The listing builds one solid part. Answer for the finished solid, in the listing's coordinates (mm). Coordinates: 2 decimals unless noted, no trailing zeros. Order: outer loops, then holes, each group sorted by start corner. A loop starts at its lowest first (then second) coordinate and runs counter-clockwise, first axis right, second up. Notation, with made-up numbers: M 14.5,-38.75 L 33.5,-38.75 A13 ccw 33.5,-22.75 Z; hole C 66.25,-25 d8. An arc over 180 degrees is marked long. One line per item, written item: value. Start each with the question number.
Q1. This flat-tipped pin is pushed along its axis until it touches: pin 1 Ø5.5 at (x, y) = (0, 60) entering from +Z. Where does it stop, or does it pass through?
Q2. Straight lines are drawn through the part: line 1 along Y through (x, z) = (0, 0.4); line 2 along Y through (x, z) = (2, 0.95); line 3 along X through (y, z) = (22.5, 1.15). For each, find the intervals that lie inside material, in ascending order. Write a range as [from, to].
Q3. The part is cut by section B-B on z = 1.3. Give the vertices of the cut face in (x, y), then the cut area to 3 significant figures.
Q4. The part is cut by section D-D on y = -62. Give the vertices of the cut face in (x, z).
Q5. The part is cut by section A-A on x = 0. Give the vertices of the cut face in (y, z), then the cut area to 3 significant figures.
Q6. The part is cut by section C-C on y = 60. Give the vertices of the cut face in (x, z), then the cut area to 3 significant figures.
```python
from build123d import *

# Parameters (mm, degrees)
SKETCH_1_W        = 40
SKETCH_1_H        = 160
EXTRUDE_1_DEPTH   = 2
CHAMFER_1_SIZE    = 2
HOLE_WIZARD_M81_D = 9


with BuildPart() as part:
    # Эскиз1 → Бобышка-Вытянуть1 (new body)
    with BuildSketch(Plane.XY):
        Rectangle(SKETCH_1_W, SKETCH_1_H)
    extrude(amount=EXTRUDE_1_DEPTH)

    # Фаска1
    chamfer_1_edges = [part.edges().sort_by_distance(p)[0] for p in [
        (20, -80, 1),
        (-20, -80, 1),
        (-20, 80, 1),
        (20, 80, 1),
    ]]
    chamfer(chamfer_1_edges, length=CHAMFER_1_SIZE)

    # Отверстие с зазором M81 (through all)
    with Locations(Plane.XY.offset(2)):
        with Locations((0, -60), (0, 60), (0, 20), (0, -20)):
            Hole(HOLE_WIZARD_M81_D / 2)


solid = part.part
```
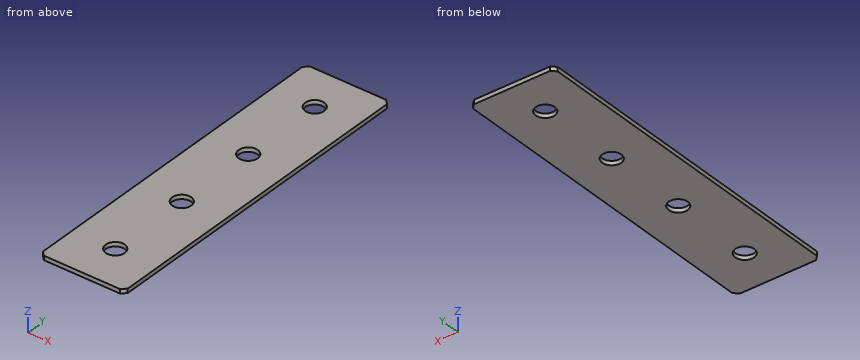
Output:
1. pin 1: passes through
2. line 1: y = [-80, -64.5], [-55.5, -24.5], [-15.5, 15.5], [24.5, 55.5], [64.5, 80]
2. line 2: y = [-80, -64.03], [-55.97, -24.03], [-15.97, 15.97], [24.03, 55.97], [64.03, 80]
2. line 3: x = [-20, -3.74], [3.74, 20]
3. outline: M -20,-78 L -18,-80 L 18,-80 L 20,-78 L 20,78 L 18,80 L -18,80 L -20,78 Z; hole C 0,-60 d9; hole C 0,-20 d9; hole C 0,20 d9; hole C 0,60 d9
3. area: 6,140 mm^2
4. outline: M -20,0 L -4.03,0 L -4.03,2 L -20,2 Z; M 4.03,0 L 20,0 L 20,2 L 4.03,2 Z
5. outline: M -80,0 L -64.5,0 L -64.5,2 L -80,2 Z; M -55.5,0 L -24.5,0 L -24.5,2 L -55.5,2 Z; M -15.5,0 L 15.5,0 L 15.5,2 L -15.5,2 Z; M 24.5,0 L 55.5,0 L 55.5,2 L 24.5,2 Z; M 64.5,0 L 80,0 L 80,2 L 64.5,2 Z
5. area: 248 mm^2
6. outline: M -20,0 L -4.5,0 L -4.5,2 L -20,2 Z; M 4.5,0 L 20,0 L 20,2 L 4.5,2 Z
6. area: 62.0 mm^2
